Source: CAD feature listing. Evaluate the final solid. Frame: model axes, mm. A direction names the side the tool comes from. Give positions to 0.01 mm unless a question says otherwise; leave off trailing zeros. Write each loop counter-clockwise with the first axis right and the second up, starting at its lowest first coordinate (ties: lowest second). Pieces come first, ordered by that corner, then holes.
```python
from build123d import *

# Parameters (mm, degrees)
BOSS_EXTRUDE1_DEPTH = 10
SKETCH2_W           = 10
SKETCH2_H           = 25.2
BOSS_EXTRUDE2_DEPTH = 150
SKETCH3_R           = 1.7
CUT_EXTRUDE1_DEPTH  = 236.69853627
CUT_EXTRUDE2_DEPTH  = 5
FILLET1_R           = 10
FILLET2_R           = 5


with BuildPart() as part:
    # Sketch1 → Boss-Extrude1 (new body)
    with BuildSketch(Plane(origin=(0, 0, 0), x_dir=(1, 0, 0), z_dir=(0, 1, 0))):
        Polygon((12.6, 12.6), (77.4, 12.6), (77.4, -12.6), (12.6, -12.6), (12.6, -77.4), (-12.6, -77.4), (-12.6, -12.6), (-77.4, -12.6), (-77.4, 12.6), (-12.6, 12.6), (-12.6, 77.4), (12.6, 77.4), align=None)
    extrude(amount=BOSS_EXTRUDE1_DEPTH)

    # Sketch2 → Boss-Extrude2 (add)
    with BuildSketch(Plane(origin=(0, 10, 0), x_dir=(1, 0, 0), z_dir=(0, 1, 0))):
        with Locations((72.4, 0)):
            Rectangle(SKETCH2_W, SKETCH2_H)
    boss_extrude2 = extrude(amount=BOSS_EXTRUDE2_DEPTH)

    # Sketch3 → Cut-Extrude1 (cut, through all)
    with BuildSketch(Plane(origin=(77.4, 0, 0), x_dir=(0, 0, -1), z_dir=(1, 0, 0))):
        with Locations((-6.3, 147.4)):
            Circle(SKETCH3_R)
        with Locations((6.3, 147.4)):
            Circle(SKETCH3_R)
    cut_extrude1 = extrude(amount=-CUT_EXTRUDE1_DEPTH, mode=Mode.SUBTRACT)

    # Sketch4 → Cut-Extrude2 (cut)
    with BuildSketch(Plane.ZY.offset(-67.4)):
        Polygon((-6.3, 143.935898385), (-3.3, 145.667949192), (-3.3, 149.132050808), (-6.3, 150.864101615), (-9.3, 149.132050808), (-9.3, 145.667949192), align=None)
        Polygon((9.3, 145.667949192), (6.3, 143.935898385), (3.3, 145.667949192), (3.3, 149.132050808), (6.3, 150.864101615), (9.3, 149.132050808), align=None)
    cut_extrude2 = extrude(amount=-CUT_EXTRUDE2_DEPTH, mode=Mode.SUBTRACT)

    # Mirror1: Boss-Extrude2, Cut-Extrude1, Cut-Extrude2 across plane
    add(boss_extrude2.mirror(Plane(origin=(0, 0, 0), x_dir=(0, 0, 1), z_dir=(1, 0, 0))))
    add(cut_extrude1.mirror(Plane(origin=(0, 0, 0), x_dir=(0, 0, 1), z_dir=(1, 0, 0))), mode=Mode.SUBTRACT)
    add(cut_extrude2.mirror(Plane(origin=(0, 0, 0), x_dir=(0, 0, 1), z_dir=(1, 0, 0))), mode=Mode.SUBTRACT)

    # Fillet1
    fillet1_edges = [part.edges().sort_by_distance(p)[0] for p in [
        (12.6, 5, 12.6),
        (-12.6, 5, 12.6),
        (-12.6, 5, -12.6),
        (12.6, 5, -12.6),
    ]]
    fillet(fillet1_edges, radius=FILLET1_R)

    # Fillet2
    fillet2_edges = [part.edges().sort_by_distance(p)[0] for p in [
        (67.4, 160, 0),
        (-67.4, 160, 0),
    ]]
    fillet(fillet2_edges, radius=FILLET2_R)


solid = part.part
```
1. Cut plane C-C, the plane x = 64. Return the cut outline in (y, z), then the cut area to 3 significant figures.
2. Mould query, pull axis Y, two halves, no side actions, for faces 1 (the flat face through (5, 10, 0)), 2 (the flat face through (-72.4, 146, -8)), 3 (the flat face through (-68, 62, 12.6)), 4 (the flat face through (-72.4, 146, 8)). Classes: +Y half, -Y half, draft (parallel to the pull), parting line (faces both ways), or undercut.
3. Cut plane B-B, the plane z = 36. Return the cut outline in (x, y).
4. Cut plane A-A, the plane y = 28. Return the cut outline in (x, z).
5. Contact query for flat-ended pins moving along their axis: P1, Ø16.5, axis at x = -53.5, y = 77.5, coming from the +Z side; P2, Ø1, axis at x = 69, y = 146.5, coming from the -Z side; P3, Ø4, axis at x = -71, y = 146.5, coming from the +Z side. Output: stop coordinate, or through.
6. Line query: L1, parallel to Z at x = 75.25, y = 147.4; L2, parallel to X at y = 90, z = -12; L3, parallel to Y at x = 76.2, z = -6.3. Output: solid intervals per line, ascending.
7. Access query for faces 5 (the cylindrical face through (68.83, 158.5, -0.18)), 6 (the flat face through (-68, 62, -12.6)), 7 (the flat face through (12.6, 5, -50)). Directions: +Z, -Z, +X, -X, +Y, -Y. A direction counts if a zero-diameter tool reaches every point of the face in a straight line with its end or side. Return the directions, or none.
Response values:
1. outline: (0, -12.6) - (10, -12.6) - (10, 12.6) - (0, 12.6) - close
1. area: 252 mm2
2. face 1: +Y half
2. face 2: undercut
2. face 3: draft
2. face 4: undercut
3. outline: (-12.6, 0) - (12.6, 0) - (12.6, 10) - (-12.6, 10) - close
4. outline: (-77.4, -12.6) - (-67.4, -12.6) - (-67.4, 12.6) - (-77.4, 12.6) - close; (67.4, -12.6) - (77.4, -12.6) - (77.4, 12.6) - (67.4, 12.6) - close
5. P1: passes through
5. P2: stops at z = -12.6
5. P3: stops at z = 12.6
6. L1: z = -12.6 to -8, -4.6 to 4.6, 8 to 12.6
6. L2: x = -77.4 to -67.4, 67.4 to 77.4
6. L3: y = 0 to 145.7, 149.1 to 160
7. face 5: +Z, -Z, +Y
7. face 6: -Z, -X, +Y, -Y
7. face 7: -Z, +X, +Y, -Y
